Here's the drawing with two shaded views (mm, measured from the low corner). I have some questions. Coordinates: 2 decimals unless noted, no trailing zeros. Order: outer loops, then holes, each group sorted by start corner. A loop starts at its lowest first (then second) coordinate and runs counter-clockwise, first axis right, second up. Notation, with made-up numbers: (28.25, 65) -> (40.25, 65) arc R18 cw to (40.25, 95) -> close; hole circle Ø6 at (7, -1). An arc over 180 degrees is marked (long way). Answer as a JSON object with one key per item and string values. Group by question number.
(1) If we mould it in two halves opening along X, with no side actions, what happens to the marked faces 1, 2, 3 and 4? For each: pulls with the +X half, pulls with the -X half, needs draft (parallel to the pull), parting line crosses it, or undercut.
(2) I want a section at C-C, the plane x = 2. List the corners of the cut face in (y, z) for me, plus the area to 3 significant figures.
(3) I want a section at D-D, the plane z = 1.3. List the corners of the cut face in (x, y) for me.
(4) I want a section at A-A, the plane z = 2.5. List the corners of the cut face in (x, y) for me.
(5) I need wall thicknesses on line 1 (X direction, y = 1.25, z = 4.2) (1 decimal); line 2 (X direction, y = 1.5, z = 3.5); line 3 (X direction, y = 5.25, z = 4.35) (1 decimal). Which ranges of each line are inside material? Lowest first, please.
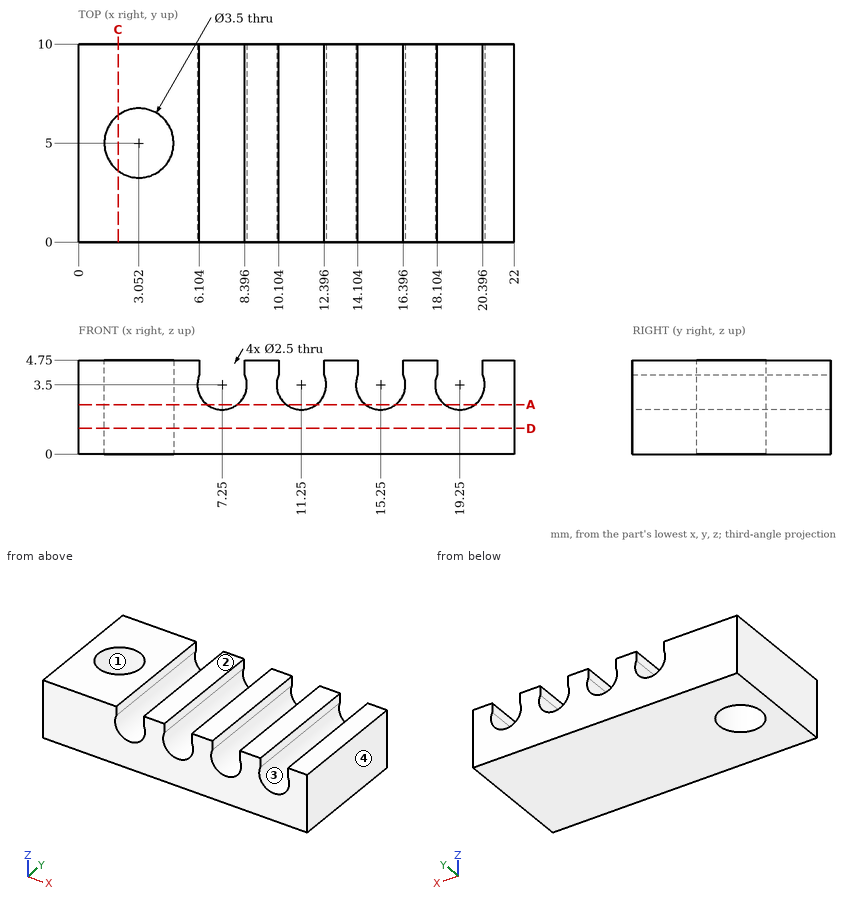
Computed values:
{
 "1": {"face 1": "undercut", "face 2": "needs draft", "face 3": "undercut", "face 4": "pulls with the +X half"},
 "2": {"outline": "(0, 0) -> (3.6, 0) -> (3.6, 4.75) -> (0, 4.75) -> close; (6.4, 0) -> (10, 0) -> (10, 4.75) -> (6.4, 4.75) -> close", "area": "34.2 mm2"},
 "3": {"outline": "(0, 0) -> (22, 0) -> (22, 10) -> (0, 10) -> close; hole circle Ø3.5 at (3.05, 5)"},
 "4": {"outline": "(0, 0) -> (6.5, 0) -> (6.5, 10) -> (0, 10) -> close; (8, 0) -> (10.5, 0) -> (10.5, 10) -> (8, 10) -> close; (12, 0) -> (14.5, 0) -> (14.5, 10) -> (12, 10) -> close; (16, 0) -> (18.5, 0) -> (18.5, 10) -> (16, 10) -> close; (20, 0) -> (22, 0) -> (22, 10) -> (20, 10) -> close; hole circle Ø3.5 at (3.05, 5)"},
 "5": {"line 1": "x = 0 to 6.1, 8.4 to 10.1, 12.4 to 14.1, 16.4 to 18.1, 20.4 to 22", "line 2": "x = 0 to 6, 8.5 to 10, 12.5 to 14, 16.5 to 18, 20.5 to 22", "line 3": "x = 0 to 1.3, 4.8 to 6.1, 8.4 to 10.1, 12.4 to 14.1, 16.4 to 18.1, 20.4 to 22"}
}
